For this review, take the finished solid that the model builds, in its own axes (mm). Face numbers are marked on the shaded views. A direction names the side the tool comes from. Give positions to 0.01 mm unless a question says otherwise; leave off trailing zeros. Loops run counter-clockwise (first coordinate to the right, second up) from the corner with the lowest first, then second, coordinate; pieces in that order, holes last.
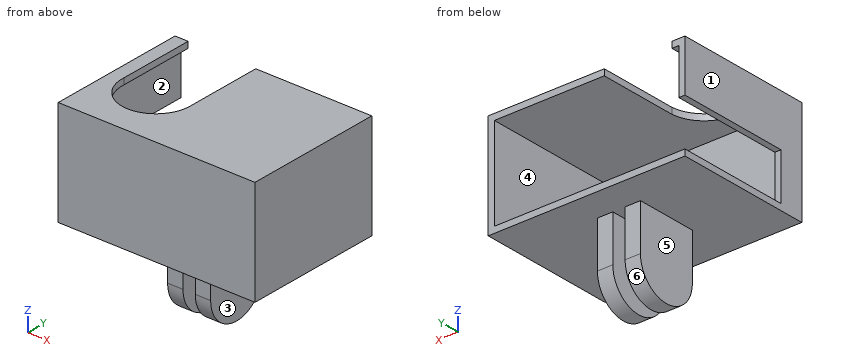
```python
from build123d import *

# Parameters (mm, degrees)
SKETCH1_W           = 64
SKETCH1_H           = 45
BOSS_EXTRUDE1_DEPTH = 34
CUT_EXTRUDE2_START  = -2
SKETCH3_W           = 60
SKETCH3_H           = 41
CUT_EXTRUDE2_DEPTH  = 27
SKETCH4_W           = 60
SKETCH4_H           = 30
CUT_EXTRUDE3_DEPTH  = 43
BOSS_EXTRUDE2_START = 2
BOSS_EXTRUDE2_DEPTH = 5
BOSS_EXTRUDE3_START = -7
BOSS_EXTRUDE3_DEPTH = 5
SKETCH10_W          = 15.255500618
SKETCH10_H          = 37
CUT_EXTRUDE5_DEPTH  = 2
SKETCH15_W          = 22
SKETCH15_H          = 26
CUT_EXTRUDE6_DEPTH  = 10
SKETCH20_R          = 11
CUT_EXTRUDE7_DEPTH  = 10


with BuildPart() as part:
    # Sketch1 → Boss-Extrude1 (new body)
    with BuildSketch(Plane.XY):
        with Locations((1.653781513, -3.994957983)):
            Rectangle(SKETCH1_W, SKETCH1_H)
    extrude(amount=BOSS_EXTRUDE1_DEPTH)

    # Sketch3 → Cut-Extrude2 (cut)
    with BuildSketch(Plane.XY.offset(34).offset(CUT_EXTRUDE2_START)):
        with Locations((1.653781513, -3.994957983)):
            Rectangle(SKETCH3_W, SKETCH3_H)
    extrude(amount=-CUT_EXTRUDE2_DEPTH, mode=Mode.SUBTRACT)

    # Sketch4 → Cut-Extrude3 (cut)
    with BuildSketch(Plane(origin=(0, 18.505042017, 0), x_dir=(1, 0, 0), z_dir=(0, 1, 0))):
        with Locations((1.653781513, -17)):
            Rectangle(SKETCH4_W, SKETCH4_H)
    extrude(amount=-CUT_EXTRUDE3_DEPTH, mode=Mode.SUBTRACT)

    # Sketch7 → Boss-Extrude2 (add)
    with BuildSketch(Plane(origin=(0, 0, 0), x_dir=(0, 0, -1), z_dir=(1, 0, 0)).offset(BOSS_EXTRUDE2_START)):
        with BuildLine():
            Line((0, 7.999642933), (15, 7.999642933))
            ThreePointArc((15, 7.999642933), (25, -2.000357067), (15, -12.000357067))
            Line((15, -12.000357067), (0, -12.000357067))
            Line((0, -12.000357067), (0, 7.999642933))
        make_face()
    extrude(amount=BOSS_EXTRUDE2_DEPTH)

    # Sketch8 → Boss-Extrude3 (add)
    with BuildSketch(Plane(origin=(0, 0, 0), x_dir=(0, 0, -1), z_dir=(1, 0, 0)).offset(BOSS_EXTRUDE3_START)):
        with BuildLine():
            Line((0, -12.000357067), (0, 7.999642933))
            Line((0, 7.999642933), (15, 7.999642933))
            ThreePointArc((15, 7.999642933), (25, -2.000357067), (15, -12.000357067))
            Line((15, -12.000357067), (0, -12.000357067))
        make_face()
    extrude(amount=BOSS_EXTRUDE3_DEPTH)

    # Sketch10 → Cut-Extrude5 (cut)
    with BuildSketch(Plane.ZY.offset(30.346218487)):
        with Locations((9.627750309, 0.005042017)):
            Rectangle(SKETCH10_W, SKETCH10_H)
    extrude(amount=-CUT_EXTRUDE5_DEPTH, mode=Mode.SUBTRACT)

    # Sketch15 → Cut-Extrude6 (cut)
    with BuildSketch(Plane.XY.offset(34)):
        with Locations((-15.092768172, 5.505042017)):
            Rectangle(SKETCH15_W, SKETCH15_H)
    extrude(amount=-CUT_EXTRUDE6_DEPTH, mode=Mode.SUBTRACT)

    # Sketch20 → Cut-Extrude7 (cut)
    with BuildSketch(Plane.XY.offset(34)):
        with Locations((-15.112148053, -6.889817492)):
            Circle(SKETCH20_R)
    extrude(amount=-CUT_EXTRUDE7_DEPTH, mode=Mode.SUBTRACT)


solid = part.part
```
Q1. Machinability: for the marked faces 4, 5 and 6, which of the approach directions +Z, -Z, +X, -X, +Y, -Y give a long, thin tool a straight path to every point of the face, cutting with its end or side? Answer none if there is none.
Answers:
face 4: +Y
face 5: -Z, -X, +Y, -Y
face 6: -Z, +X, -X
Q2. For pin 1 Ø5.5 at (x, z) = (3.5, -5) entering from -Y; pin 2 Ø3 at (y, z) = (-1, 4.5) entering from -X; pin 3 Ø16 at (y, z) = (1.5, -9.5) entering from -X, all flat-tipped, find the tip position at first contact; note any pin that passes through.
Answers:
pin 1: stops at y = -12
pin 2: stops at x = 31.65
pin 3: stops at x = -7
Q3. Consider section C-C on x = 17.5. Give the boundary of the cut face in (y, z).
Answers:
outline: (-26.49, 0) - (18.51, 0) - (18.51, 2) - (-24.49, 2) - (-24.49, 32) - (18.51, 32) - (18.51, 34) - (-26.49, 34) - close
Q4. For probe 1 along Z at (x, y) = (3, 10); probe 2 along X at (y, z) = (8, 30.5); probe 3 along X at (y, z) = (4, -21), list the stretches that pass through material, from the lowest coordinate up.
Answers:
probe 1: z = 0 to 2, 32 to 34
probe 2: x = -30.35 to -28.35, 31.65 to 33.65
probe 3: x = -7 to -2, 2 to 7
Q5. Consider section A-A on z = -12.5. Give the boundary of the cut face in (x, y), plus the area to 3 significant figures.
Answers:
outline: (-7, -12) - (-2, -12) - (-2, 8) - (-7, 8) - close; (2, -12) - (7, -12) - (7, 8) - (2, 8) - close
area: 200 mm2
Q6. Mouldability with a two-part tool opening along X and no side actions: class the marked faces 1, 2 and 3 as +X half, -X half, draft (parallel to the pull), parting line (faces both ways), or undercut.
Answers:
face 1: -X half
face 2: undercut
face 3: +X half
Q7. Consider section D-D on z = 5.5. Give the boundary of the cut face in (x, y).
Answers:
outline: (-30.35, -26.49) - (33.65, -26.49) - (33.65, 18.51) - (31.65, 18.51) - (31.65, -24.49) - (-28.35, -24.49) - (-28.35, -18.49) - (-30.35, -18.49) - close
Q8. Consider section B-B on y = -9. Give the boundary of the cut face in (x, z).
Answers:
outline: (-30.35, 0) - (-7, 0) - (-7, -22.14) - (-2, -22.14) - (-2, 0) - (2, 0) - (2, -22.14) - (7, -22.14) - (7, 0) - (33.65, 0) - (33.65, 34) - (-4.32, 34) - (-4.32, 32) - (31.65, 32) - (31.65, 2) - (-30.35, 2) - close; (-30.35, 17.26) - (-28.35, 17.26) - (-28.35, 32) - (-25.91, 32) - (-25.91, 34) - (-30.35, 34) - close
